Source: three-view drawing plus pictorial views. Frame: mm from the lowest corner of the part. A direction names the side the tool comes from. Give positions to 0.01 mm unless a question says otherwise; leave off trailing zeros. Order: outer loops, then holes, each group sorted by start corner. A loop starts at its lowest first (then second) coordinate and runs counter-clockwise, first axis right, second up. Notation, with made-up numbers: (60.25, -7) -> (94.25, -7) arc R33 cw to (94.25, 31) -> close; hole circle Ø6 at (-30, 37.5). An arc over 180 degrees is marked (long way). One line per question, with ' | ' between items.
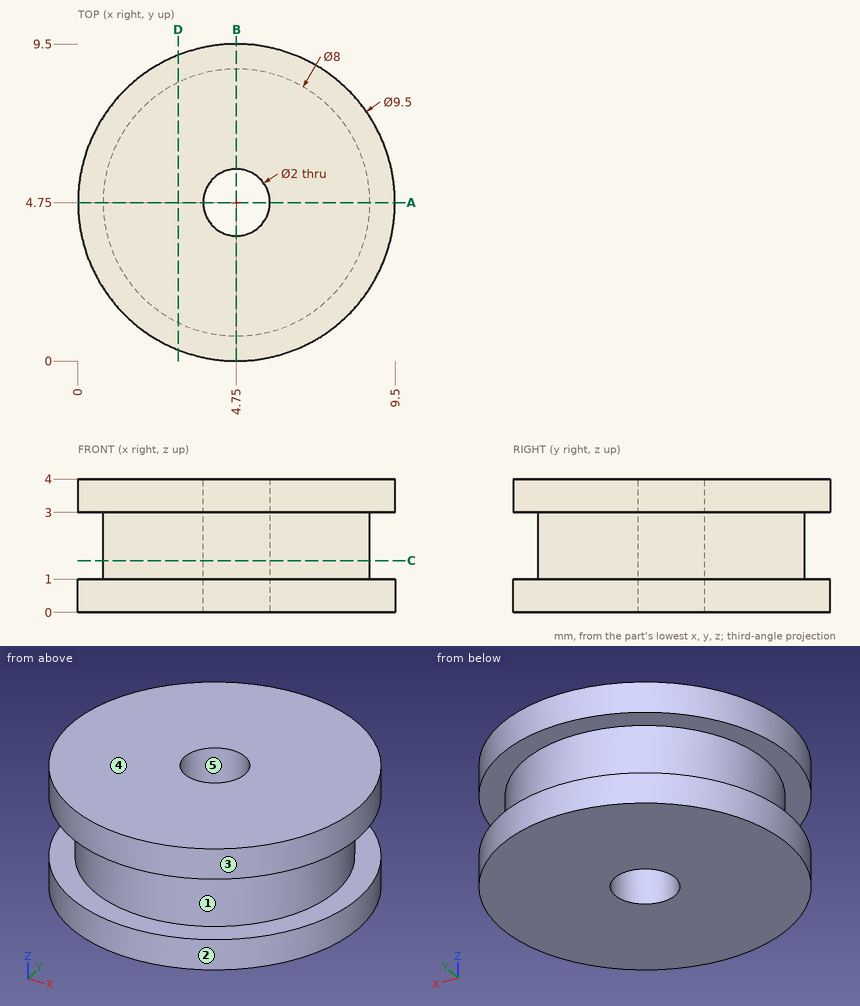
1) Contact query for a flat-ended pin moving along its axis: pin 1 Ø5 at (x, y) = (4, 2.5) entering from -Z. Output: stop coordinate, or through.
Check result:
pin 1: stops at z = 0
2) Section A-A on y = 4.75. Return loops of the section in (x, z), plus the area to 3 significant figures.
Check result:
outline: (0, 0) -> (3.75, 0) -> (3.75, 4) -> (0, 4) -> (0, 3) -> (0.75, 3) -> (0.75, 1) -> (0, 1) -> close; (5.75, 0) -> (9.5, 0) -> (9.5, 1) -> (8.75, 1) -> (8.75, 3) -> (9.5, 3) -> (9.5, 4) -> (5.75, 4) -> close | area: 27.0 mm^2
3) Section C-C on z = 1.55. Return loops of the section in (x, y).
Check result:
outline: circle Ø8 at (4.75, 4.75); hole circle Ø2 at (4.75, 4.75)
4) Section D-D on x = 3. Return loops of the section in (y, z), plus the area to 3 significant figures.
Check result:
outline: (0.33, 0) -> (9.17, 0) -> (9.17, 1) -> (8.35, 1) -> (8.35, 3) -> (9.17, 3) -> (9.17, 4) -> (0.33, 4) -> (0.33, 3) -> (1.15, 3) -> (1.15, 1) -> (0.33, 1) -> close | area: 32.1 mm^2
5) Material intervals for probe 1 along Z at (x, y) = (8.5, 6.5); probe 2 along Y at (x, z) = (4.75, 1.15); probe 3 along Y at (x, z) = (4, 0.9), sorted ascending. Write a range as from..to.
Check result:
probe 1: z = 0..1, 3..4 | probe 2: y = 0.75..3.75, 5.75..8.75 | probe 3: y = 0.06..4.09, 5.41..9.44
6) Set-up query: the marked faces 1 and 2. Return all of +Z, -Z, +X, -X, +Y, -Y with unobstructed straight access to the full face (end or side cutting, diameter ignored); none if empty.
Check result:
face 1: none | face 2: +Z, -Z
7) Pull-direction query (X, two-part tool) for the marked faces 3, 4 and 5; classes: +X half, -X half, draft (parallel to the pull), parting line (faces both ways), or undercut.
Check result:
face 3: parting line | face 4: draft | face 5: undercut
